Answer from the drawing. Dimensions are ordinates in mm from the lowest x, y and z of the part. Round coordinates to 2 decimals unless told otherwise and drop trailing zeros. Loops run counter-clockwise (first coordinate to the right, second up) from the corner with the lowest first, then second, coordinate; pieces in that order, holes last.
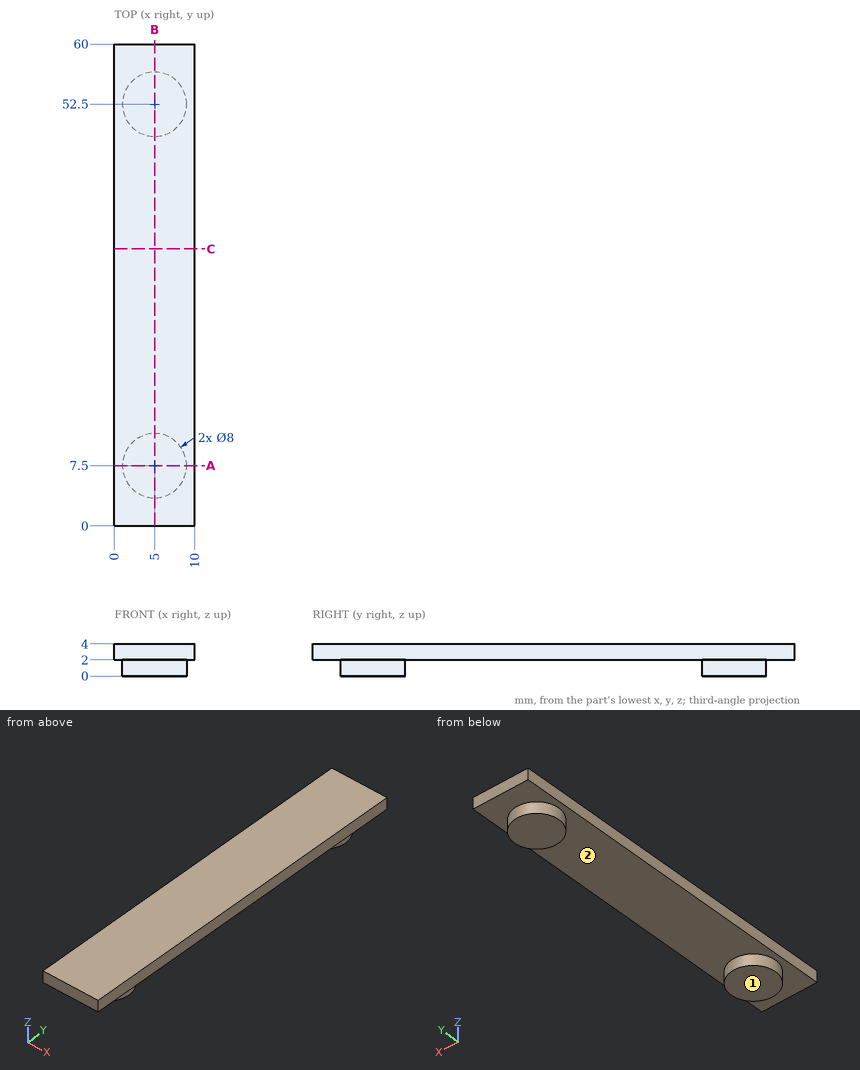
Item 1: Section C-C, the plane y = 34.5 is taken. Give the vertices of the cut face in (x, z), plus the area to 3 significant figures.
Item 2: This flat-tipped pin is pushed along its axis until it touches: P1, Ø4, axis at x = 4, y = 18.5, coming from the -Z side. Where does it stop, or does it pass through?
Item 3: Section A-A, the plane y = 7.5 is taken. Give the vertices of the cut face in (x, z), plus the area to 3 significant figures.
Item 4: Section B-B, the plane x = 5 is taken. Give the vertices of the cut face in (y, z).
Item 5: Determine the mould class of the marked faces 1 and 2 for opening direction Y: pulls with the +Y half, pulls with the -Y half, needs draft (parallel to the pull), parting line crosses it, or undercut.
Item 6: Straight lines are drawn through the part: line 1 (Z direction, x = 8, y = 55.5); line 2 (Y direction, x = 2.5, z = 1.05); line 3 (Y direction, x = 4.75, z = 0.45). For each, find the intervals that lie inside material, in ascending order.
Answer below:
1. outline: (0, 2) - (10, 2) - (10, 4) - (0, 4) - close
1. area: 20.0 mm2
2. P1: stops at z = 2
3. outline: (0, 2) - (1, 2) - (1, 0) - (9, 0) - (9, 2) - (10, 2) - (10, 4) - (0, 4) - close
3. area: 36.0 mm2
4. outline: (0, 2) - (3.5, 2) - (3.5, 0) - (11.5, 0) - (11.5, 2) - (48.5, 2) - (48.5, 0) - (56.5, 0) - (56.5, 2) - (60, 2) - (60, 4) - (0, 4) - close
5. face 1: needs draft
5. face 2: undercut
6. line 1: z = 2 to 4
6. line 2: y = 4.38 to 10.62, 49.38 to 55.62
6. line 3: y = 3.51 to 11.49, 48.51 to 56.49
